Check sheet for the modelled part. Datum: model origin and axes. Units: mm. A direction names the side the tool comes from. Round coordinates to 2 decimals unless told otherwise and drop trailing zeros. Order: outer loops, then holes, each group sorted by start corner. A loop starts at its lowest first (then second) coordinate and runs counter-clockwise, first axis right, second up.
(1) Sectioned sample at C-C, the plane z = 6. Enter the section's corners in (x, y), and give its area (3 significant figures).
(2) Mould release check, pull along Z, two halves, no side actions. Record for faces 1 (the flat face through (2, -2, 0)), 2 (the cylindrical face through (-3.469, 1.059, 2.947)), 3 (the flat face through (-4, 0, 4.5)): released by +Z, released by -Z, zero draft, split by the parting line, or undercut.
(3) Tool access check on faces 4 (the cylindrical face through (3.233, -1.341, 6.62)), 5 (the cylindrical face through (2.5, 0.1, 4.3)). Record the directions out of +Z, -Z, +X, -X, +Y, -Y that give a thin tool (end or side, any length) a straight path to the whole face; none if there is none.
(4) Thickness scan on probe 1 along Y at (x, z) = (0, 5.5); probe 2 along Y at (x, z) = (0, 2.25); probe 3 along Z at (x, y) = (-0.25, -3.75). Record the ranges inside material, lowest first.
(5) Sectioned sample at B-B, the plane y = -1.75. Enter the section's corners in (x, z), and give its area (3 significant figures).
(6) Sectioned sample at D-D, the plane y = 4. Enter the section's corners in (x, z).
(7) Depth check by flat-ended pin: pin 1 (5 mm diameter, centred on y = 2.5, z = 7.5, fed in from -X); pin 2 (1.5 mm diameter, centred on x = -3, z = 6, fed in from +Y). Enter the tip coordinate at first touch or a pass-through.
(8) Sectioned sample at A-A, the plane x = 0. Enter the section's corners in (y, z).
```python
from build123d import *

# Parameters (mm, degrees)
ESQUISSE1_R             = 4.75
BOSS_EXTRU_1_DEPTH      = 8.8
ENL_V_START             = -4.3
ESQUISSE2_R             = 4.75
ESQUISSE2_R_2           = 3.5
ENL_V_MAT_EXTRU_1_DEPTH = 4.3
ESQUISSE3_R             = 2.5
ENL_V_MAT_EXTRU_2_DEPTH = 12.070907822
ESQUISSE5_R             = 1.25
ENL_V_MAT_EXTRU_3_DEPTH = 5


with BuildPart() as part:
    # Esquisse1 → Boss.-Extru.1 (new body)
    with BuildSketch(Plane.XY):
        Circle(ESQUISSE1_R)
    extrude(amount=BOSS_EXTRU_1_DEPTH)

    # Esquisse2 → Enlèv. mat.-Extru.1 (cut)
    with BuildSketch(Plane.XY.offset(8.8).offset(ENL_V_START)):
        Circle(ESQUISSE2_R)
        Circle(ESQUISSE2_R_2, mode=Mode.SUBTRACT)
    extrude(amount=ENL_V_MAT_EXTRU_1_DEPTH, mode=Mode.SUBTRACT)

    # Esquisse3 → Enlèv. mat.-Extru.2 (cut, through all)
    with BuildSketch(Plane(origin=(0, 0, 0), x_dir=(-1, 0, 0), z_dir=(0, 0, -1))):
        Circle(ESQUISSE3_R)
    extrude(amount=-ENL_V_MAT_EXTRU_2_DEPTH, mode=Mode.SUBTRACT)

    # Esquisse5 → Enlèv. mat.-Extru.3 (cut)
    with BuildSketch(Plane(origin=(-4.749906239, 0.029844934, 2.25), x_dir=(0, 0, 1), z_dir=(-0.9999802608561372, 0.006283143965558953, 0))):
        with Locations(Location((0, 0, 0), (0, 0, 358.631878995))):
            Circle(ESQUISSE5_R)
    extrude(amount=-ENL_V_MAT_EXTRU_3_DEPTH, mode=Mode.SUBTRACT)


solid = part.part
```
Derived:
1. outline: circle Ø7 at (0, 0); hole circle Ø5 at (0, 0)
1. area: 18.8 mm2
2. face 1: released by -Z
2. face 2: undercut
2. face 3: released by +Z
3. face 4: +Z
3. face 5: +Z, -Z
4. probe 1: y = -3.5 to -2.5, 2.5 to 3.5
4. probe 2: y = -4.75 to -2.5, 2.5 to 4.75
4. probe 3: z = 0 to 4.5
5. outline: (-4.42, 0) - (-1.79, 0) - (-1.79, 8.8) - (-3.03, 8.8) - (-3.03, 4.5) - (-4.42, 4.5) - close; (1.79, 0) - (4.42, 0) - (4.42, 4.5) - (3.03, 4.5) - (3.03, 8.8) - (1.79, 8.8) - close
5. area: 34.4 mm2
6. outline: (-2.56, 0) - (2.56, 0) - (2.56, 4.5) - (-2.56, 4.5) - close
7. pin 1: stops at x = -3.5
7. pin 2: stops at y = 2.68
8. outline: (-4.75, 0) - (-2.5, 0) - (-2.5, 8.8) - (-3.5, 8.8) - (-3.5, 4.5) - (-4.75, 4.5) - close; (2.5, 0) - (4.75, 0) - (4.75, 4.5) - (3.5, 4.5) - (3.5, 8.8) - (2.5, 8.8) - close
